Geometry: final body of the model. Coordinates: model frame, mm. A direction names the side the tool comes from. Round coordinates to 2 decimals unless told otherwise and drop trailing zeros. Loops run counter-clockwise (first coordinate to the right, second up) from the corner with the lowest first, then second, coordinate; pieces in that order, holes last. Notation, with made-up numbers: (-19, 74) - (11, 74) arc R19 cw to (11, 89) - close; hole circle Ø3 at (-0.5, 55). An arc over 180 degrees is marked (long way). Answer as CSV lines item,"result".
from build123d import *

# Parameters (mm, degrees)
F1_DEPTH  = 3
F3_D      = 7
F4_R      = 0.2
F5_DEPTH  = 12.5
F6_W      = 12
F6_H      = 40
F7_DEPTH  = 12
F8_W      = 0.2
F8_H      = 10
F9_DEPTH  = 12
F10_R     = 0.25
F11_DEPTH = 25
F12_R     = 1.9
F13_DEPTH = 14
F14_R     = 2.5392284098
F15_DEPTH = 7.5
F16_R     = 3.75
F17_DEPTH = 4


with BuildPart() as f1:
    # F0 (on Top) → F1 (new body)
    with BuildSketch(Plane.XY):
        with BuildLine():
            Line((42.5, 5), (42.5, -5))
            Line((42.5, -5), (36.1522351233, -5))
            ThreePointArc((36.1522351233, -5), (45.1458596679, -7.635020992), (50.5804776424, 0))
            ThreePointArc((50.5804776424, 0), (45.1458596679, 7.635020992), (36.1522351233, 5))
            Line((36.1522351233, 5), (42.5, 5))
        make_face()
        with BuildLine():
            ThreePointArc((-36.1522351233, 5), (-50.5804776424, 0), (-36.1522351233, -5))
            Line((-36.1522351233, -5), (-42.5, -5))
            Line((-42.5, -5), (-42.5, 5))
            Line((-42.5, 5), (-36.1522351233, 5))
        make_face()
        with BuildLine():
            Line((36.1522351233, -5), (42.5, -5))
            Line((42.5, -5), (42.5, 5))
            Line((42.5, 5), (36.1522351233, 5))
            ThreePointArc((36.1522351233, 5), (34.4195223576, 0), (36.1522351233, -5))
        make_face()
        with BuildLine():
            Line((-36.1522351233, -5), (36.1522351233, -5))
            ThreePointArc((36.1522351233, -5), (34.4195223576, 0), (36.1522351233, 5))
            Line((36.1522351233, 5), (-36.1522351233, 5))
            ThreePointArc((-36.1522351233, 5), (-34.864979008, 2.6458596679), (-34.4195223576, 0))
            ThreePointArc((-34.4195223576, 0), (-34.864979008, -2.6458596679), (-36.1522351233, -5))
        make_face()
        with BuildLine():
            Line((-42.5, -5), (-36.1522351233, -5))
            ThreePointArc((-36.1522351233, -5), (-34.864979008, -2.6458596679), (-34.4195223576, 0))
            ThreePointArc((-34.4195223576, 0), (-34.864979008, 2.6458596679), (-36.1522351233, 5))
            Line((-36.1522351233, 5), (-42.5, 5))
            Line((-42.5, 5), (-42.5, -5))
        make_face()
    extrude(amount=F1_DEPTH)

    # F3 (through all)
    with Locations(Plane.XY.offset(3)):
        with Locations((-42.5, 0), (42.5, 0)):
            Hole(F3_D / 2)

    # F4 (on Front) → F5 (cut, symmetric)
    with BuildSketch(Plane.XZ):
        with Locations((0, 21.0996698588)):
            Circle(F4_R)
    extrude(amount=F5_DEPTH, both=True, mode=Mode.SUBTRACT)

    # F6 (on Top) → F7 (join)
    with BuildSketch(Plane.XY):
        Rectangle(F6_W, F6_H)
    extrude(amount=F7_DEPTH)

    # F8 (on Top) → F9 (cut)
    with BuildSketch(Plane.XY):
        Rectangle(F8_W, F8_H)
    extrude(amount=F9_DEPTH, mode=Mode.SUBTRACT)

    # F10 (on Front) → F11 (cut, symmetric)
    with BuildSketch(Plane.XZ):
        with Locations((0, 6)):
            Circle(F10_R)
    extrude(amount=F11_DEPTH, both=True, mode=Mode.SUBTRACT)

    # F12 (on face) → F13 (cut)
    with BuildSketch(Plane.XZ.offset(20)):
        with Locations((0, 6)):
            Circle(F12_R)
    extrude(amount=-F13_DEPTH, mode=Mode.SUBTRACT)

    # F14 (on face) → F15 (cut)
    with BuildSketch(Plane.XZ.offset(20)):
        with Locations((0, 6)):
            Circle(F14_R)
    extrude(amount=-F15_DEPTH, mode=Mode.SUBTRACT)

    # F16 (on face) → F17 (cut)
    with BuildSketch(Plane.XZ.offset(20)):
        with Locations((0, 6)):
            Circle(F16_R)
    extrude(amount=-F17_DEPTH, mode=Mode.SUBTRACT)


solid = f1.part
(1) Access query for faces 4 (the face through (-21, 5, 1)), 5 (the face through (-21, -5, 1)), 6 (the face through (28, 0, 3)), 7 (the face through (-0.81, -18.03, 2.34)). Directions: +Z, -Z, +X, -X, +Y, -Y. A direction counts if a zero-diameter tool reaches every point of the face in a straight line with its end or side. Return the directions, or none.
Findings below:
face 4,"+Z, -Z, +Y"
face 5,"+Z, -Z, -Y"
face 6,"+Z, +X, +Y, -Y"
face 7,"-Y"
(2) Material intervals for line 1 along Y through (x, z) = (42.5, 1.55); line 2 along Z through (x, y) = (0, -13.35); line 3 along Z through (x, y) = (0, -18.7), sorted ascending.
Findings below:
line 1,"-8.08 to -3.5, 3.5 to 8.08"
line 2,"0 to 3.46, 8.54 to 12"
line 3,"0 to 2.25, 9.75 to 12"
(3) Section B-B (y = 1). Output: boundary loops of the cut face in (x, z), and give its area (3 significant figures).
Findings below:
outline,"(-50.52, 0) - (-45.85, 0) - (-45.85, 3) - (-50.52, 3) - close; (-39.15, 0) - (-0.1, 0) - (-0.1, 5.77) arc R0.25 cw to (-0.1, 6.23) - (-0.1, 12) - (-6, 12) - (-6, 3) - (-39.15, 3) - close; (0.1, 0) - (39.15, 0) - (39.15, 3) - (6, 3) - (6, 12) - (0.1, 12) - (0.1, 6.23) arc R0.25 cw to (0.1, 5.77) - close; (45.85, 0) - (50.52, 0) - (50.52, 3) - (45.85, 3) - close"
area,"368 mm2"
(4) Section C-C (x = -30). Output: boundary loops of the cut face in (y, z), and give its area (3 significant figures).
Findings below:
outline,"(-5, 0) - (5, 0) - (5, 3) - (-5, 3) - close"
area,"30.0 mm2"
(5) Pin query (flat end, axial travel): P1, Ø1.7, axis at y = 2.5, z = 9.5, coming from the +X side; P2, Ø5, axis at y = -7, z = 3, coming from the +X side; P3, Ø1.5, axis at y = -13.5, z = 7, coming from the -X side. Return the tip coordinate at first contact, or that it passes through.
Findings below:
P1,"x = 6"
P2,"x = 49.21"
P3,"x = -6"
(6) Section A-A (x = -42.5). Output: boundary loops of the cut face in (y, z), and give its area (3 significant figures).
Findings below:
outline,"(-8.08, 0) - (-3.5, 0) - (-3.5, 3) - (-8.08, 3) - close; (3.5, 0) - (8.08, 0) - (8.08, 3) - (3.5, 3) - close"
area,"27.5 mm2"
(7) Draft query along Z for faces 1 (the face through (0, -16, 9)), 2 (the face through (0, 20, 5)), 3 (the face through (-29, 0, 3)). Return one class per face: pulls with the +Z half, pulls with the -Z half, needs draft (parallel to the pull), parting line crosses it, or undercut.
Findings below:
face 1,"undercut"
face 2,"needs draft"
face 3,"pulls with the +Z half"
